from build123d import *

# Parameters (mm, degrees)
BOSS_EXTRUDE1_DEPTH            = 30
HOLE1_D                        = 5.4
HOLE1_CBORE_D                  = 6.2
HOLE1_CBORE_DEPTH              = 1
CHAMFER1_SIZE2                 = 0.4
CHAMFER1_SIZE                  = 1
SKETCH5_W                      = 69.5
SKETCH5_H                      = 104.5
BOSS_EXTRUDE2_DEPTH            = 12.35
CBORE_FOR_M4_SHCS1_D           = 4.8
CBORE_FOR_M4_SHCS1_CBORE_D     = 8
CBORE_FOR_M4_SHCS1_CBORE_DEPTH = 4


with BuildPart() as part:
    # Sketch1 → Boss-Extrude1 (new body)
    with BuildSketch(Plane.XY):
        Polygon((-7.3, 0.3), (-7.3, 7.875735931), (-13.3, 13.875735931), (-13.3, 16.3), (13.3, 16.3), (13.3, 13.875735931), (7.3, 7.875735931), (7.3, 0.3), (23, 0.3), (23, 28.65), (-23, 28.65), (-23, 0.3), align=None)
    extrude(amount=BOSS_EXTRUDE1_DEPTH)

    # Hole1 (through all)
    with Locations(Plane(origin=(0, 28.65, 0), x_dir=(1, 0, 0), z_dir=(0, 1, 0))):
        with Locations((0, -20)):
            CounterBoreHole(HOLE1_D / 2, HOLE1_CBORE_D / 2, HOLE1_CBORE_DEPTH)

    # Chamfer1
    chamfer1_edges = [part.edges().sort_by_distance(p)[0] for p in [
        (-3.1, 27.65, 20),
    ]]
    chamfer1_side = [part.faces().sort_by_distance(p)[0] for p in [
        (-3.1, 27.658, 20),
    ]]
    chamfer(chamfer1_edges, length=CHAMFER1_SIZE - 0.0001, length2=CHAMFER1_SIZE2 - 0.0001, reference=chamfer1_side[0])  # a hair under: the kernel refuses the full size

    # Sketch5 → Boss-Extrude2 (add)
    with BuildSketch(Plane(origin=(0, 28.65, 0), x_dir=(1, 0, 0), z_dir=(0, 1, 0))):
        with Locations((0, 52.25)):
            Rectangle(SKETCH5_W, SKETCH5_H)
    extrude(amount=-BOSS_EXTRUDE2_DEPTH)

    # CBORE for M4 SHCS1 (through all)
    with Locations(Plane(origin=(0, 16.3, 0), x_dir=(-1, 0, 0), z_dir=(0, -1, 0))):
        with Locations((-20.5, 88.75), (20.5, 88.75), (-20.5, 15.75), (20.5, 15.75)):
            CounterBoreHole(CBORE_FOR_M4_SHCS1_D / 2, CBORE_FOR_M4_SHCS1_CBORE_D / 2, CBORE_FOR_M4_SHCS1_CBORE_DEPTH)


solid = part.part
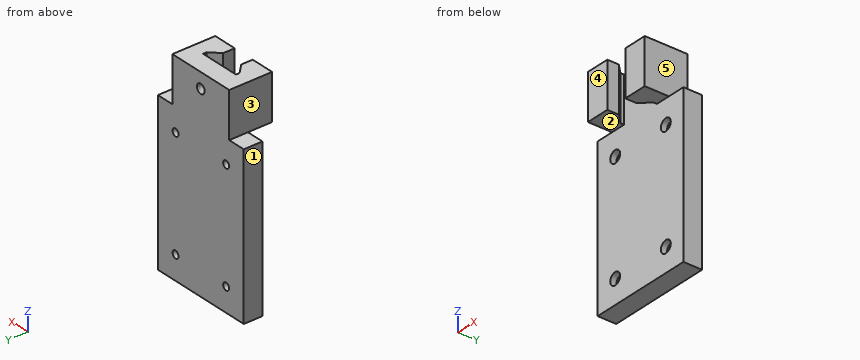
Work out the finished part from the listing and answer in its coordinate system (mm). Face numbers are marked on the shaded views. A direction names the side the tool comes from. Give positions to 0.01 mm unless a question says otherwise; leave off trailing zeros. Loops run counter-clockwise (first coordinate to the right, second up) from the corner with the lowest first, then second, coordinate; pieces in that order, holes last. Notation, with made-up numbers: (-13.5, -14.5) -> (-6.5, -14.5) arc R17 cw to (-6.5, 10.5) -> close; hole circle Ø11 at (48, 66). An arc over 180 degrees is marked (long way). Use a Markdown table: item, result. Add a question column.
1) Which of the six approach directions +Z, -Z, +X, -X, +Y, -Y give full straight-line access (tool end or side, diameter ignored) to the marked faces 1, 2, 3, 4 and 5?
2) The part is cut by section D-D, the plane x = 20.5. Determine the outline of the cut face in (y, z).
3) The part is cut by section A-A, the plane y = 3.75. Determine the outline of the cut face in (x, z), plus the area to 3 significant figures.
4) Consider line 1 along Z through (x, y) = (-20.5, 18.6); line 2 along Z through (x, y) = (20.5, 25.75); line 3 along X through (y, z) = (23.5, -88.75). Determine where each line is inside the solid, lowest interval first.
5) The part is cut by section C-C, the plane z = -88.75. Determine the outline of the cut face in (x, y), plus the area to 3 significant figures.
6) Each of these flat-tipped pins is pushed along its axis until it touches: P1, Ø5, axis at x = 20.5, z = -88.75, coming from the -Y side; P2, Ø8, axis at x = -14, y = 10.5, coming from the -Z side; P3, Ø10.5, axis at x = -20.5, z = -15.75, coming from the -Y side; P4, Ø4.5, axis at x = 0, z = 20, coming from the +Y side. Where does it stop, or does it pass through?
Reported:
| question | item | result |
|---|---|---|
| 1 | face 1 | +Z, -Z, -X, +Y, -Y |
| 1 | face 2 | -Z, +X, -X, -Y |
| 1 | face 3 | +Z, -X, +Y, -Y |
| 1 | face 4 | +Z, -Z, +X, -X, -Y |
| 1 | face 5 | +Z, +X, +Y, -Y |
| 2 | outline | (0.3, 0) -> (16.3, 0) -> (16.3, -11.75) -> (20.3, -11.75) -> (20.3, -13.35) -> (28.65, -13.35) -> (28.65, 30) -> (0.3, 30) -> close; (16.3, -104.5) -> (28.65, -104.5) -> (28.65, -91.15) -> (20.3, -91.15) -> (20.3, -92.75) -> (16.3, -92.75) -> close; (16.3, -84.75) -> (20.3, -84.75) -> (20.3, -86.35) -> (28.65, -86.35) -> (28.65, -18.15) -> (20.3, -18.15) -> (20.3, -19.75) -> (16.3, -19.75) -> close |
| 3 | outline | (-23, 0) -> (-7.3, 0) -> (-7.3, 30) -> (-23, 30) -> close; (7.3, 0) -> (23, 0) -> (23, 30) -> (7.3, 30) -> close |
| 3 | area | 942 mm^2 |
| 4 | line 1 | z = -104.5 to -92.75, -84.75 to -19.75, -11.75 to 30 |
| 4 | line 2 | z = -104.5 to -91.15, -86.35 to -18.15, -13.35 to 30 |
| 4 | line 3 | x = -34.75 to -22.9, -18.1 to 18.1, 22.9 to 34.75 |
| 5 | outline | (-34.75, 16.3) -> (-24.5, 16.3) -> (-24.5, 20.3) -> (-22.9, 20.3) -> (-22.9, 28.65) -> (-34.75, 28.65) -> close; (-18.1, 20.3) -> (-16.5, 20.3) -> (-16.5, 16.3) -> (16.5, 16.3) -> (16.5, 20.3) -> (18.1, 20.3) -> (18.1, 28.65) -> (-18.1, 28.65) -> close; (22.9, 20.3) -> (24.5, 20.3) -> (24.5, 16.3) -> (34.75, 16.3) -> (34.75, 28.65) -> (22.9, 28.65) -> close |
| 5 | area | 714 mm^2 |
| 6 | P1 | stops at y = 20.3 |
| 6 | P2 | stops at z = 0 |
| 6 | P3 | stops at y = 16.3 |
| 6 | P4 | passes through |
